Study the drawing (mm; zero at the part's minimum x, y, z) and answer. Round coordinates to 2 decimals unless told otherwise and drop trailing zeros. Write each loop counter-clockwise with the first axis right and the second up, starting at its lowest first coordinate (ties: lowest second). Pieces come first, ordered by that corner, then holes.
(1) A cutting plane is placed at A-A, the plane z = 6.25. Give the vertices of the cut face in (x, y).
(2) A cutting plane is placed at C-C, the plane x = 66. Give the vertices of the cut face in (y, z), and give its area (3 significant figures).
(3) Find the intervals of material crossed by probe 1 along Y at (x, z) = (2.5, 2.75); probe 2 along X at (y, z) = (2.5, 2); probe 3 along Y at (x, z) = (124, 2.25), in increasing order.
(4) The mould has two halves that part along Y. Classify the marked faces 1 and 2: +Y half, -Y half, draft (parallel to the pull), parting line (faces both ways), or undercut.
(5) Each of these flat-tipped pins is pushed along its axis until it touches: pin 1 Ø4 at (x, y) = (2.5, 2.5) entering from +Z; pin 2 Ø12 at (x, y) = (92, 12.5) entering from -Z. Where does it stop, or does it pass through?
(6) A cutting plane is placed at B-B, the plane y = 68. Give the vertices of the cut face in (x, z).
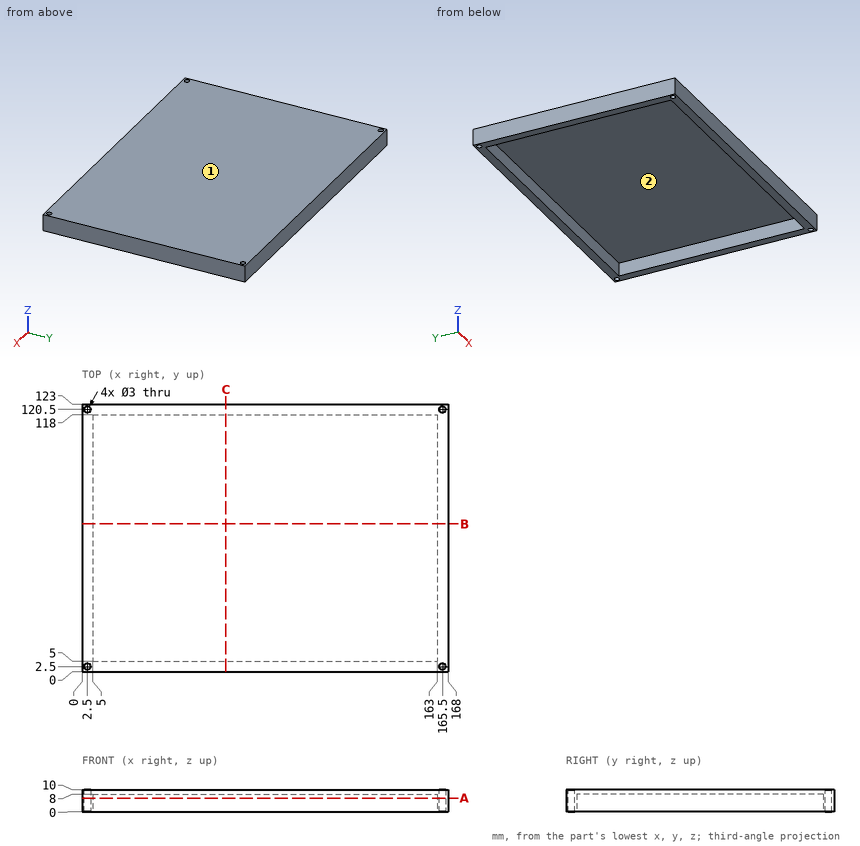
Solutions:
1. outline: (0, 0) - (168, 0) - (168, 123) - (0, 123) - close; hole circle Ø3 at (2.5, 2.5); hole circle Ø3 at (2.5, 120.5); hole (5, 5) - (163, 5) - (163, 118) - (5, 118) - close; hole circle Ø3 at (165.5, 2.5); hole circle Ø3 at (165.5, 120.5)
2. outline: (0, 0) - (5, 0) - (5, 8) - (118, 8) - (118, 0) - (123, 0) - (123, 10) - (0, 10) - close
2. area: 326 mm2
3. probe 1: y = 0 to 1, 4 to 119, 122 to 123
3. probe 2: x = 0 to 1, 4 to 164, 167 to 168
3. probe 3: y = 0 to 5, 118 to 123
4. face 1: draft
4. face 2: undercut
5. pin 1: stops at z = 10
5. pin 2: stops at z = 8
6. outline: (0, 0) - (5, 0) - (5, 8) - (163, 8) - (163, 0) - (168, 0) - (168, 10) - (0, 10) - close
